Verification items for the finished model (mm, model axes). Give positions to 0.01 mm unless a question says otherwise; leave off trailing zeros. Loops run counter-clockwise (first coordinate to the right, second up) from the corner with the lowest first, then second, coordinate; pieces in that order, holes last. Notation, with made-up numbers: (9.25, 84) - (54.25, 84) arc R15 cw to (54.25, 95) - close; hole circle Ø4 at (14, 42). An arc over 180 degrees is marked (long way). One line per question, with ' | ' between items. Start each with the question number.
1. Thickness scan on line 1 along Y through (x, z) = (170, 0.9); line 2 along Y through (x, z) = (4, 1.7); line 3 along Y through (x, z) = (80, 2.7). Record the ranges inside material, lowest first. Write a range as from..to.
2. Section check B-B, the plane y = 5.5. Enter the section's corners in (x, z), then the cut area to 3 significant figures.
3. Section check C-C, the plane z = 2.2. State how many separate pieces and enclosed holes the cut face has, then the cut area to 3 significant figures.
4. Section check A-A, the plane x = 134.5. Enter the section's corners in (y, z).
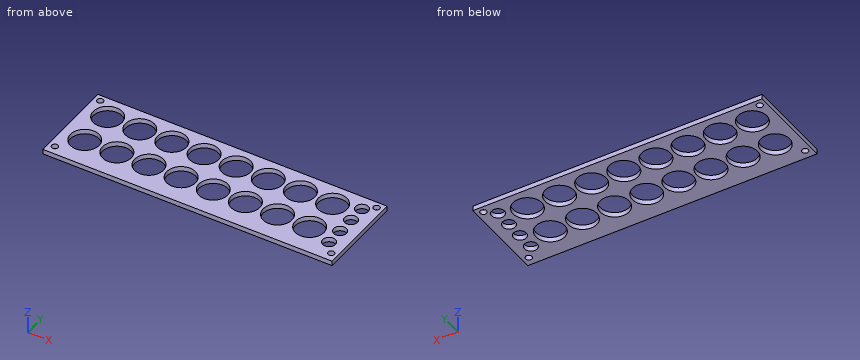
from build123d import *

# Parameters (mm, degrees)
CYLINDER023_R     = 2
CYLINDER023_DEPTH = 3
CYLINDER022_R     = 2
CYLINDER022_DEPTH = 3
CYLINDER021_R     = 2
CYLINDER021_DEPTH = 3
CYLINDER020_R     = 2
CYLINDER020_DEPTH = 3
CYLINDER019_R     = 4
CYLINDER019_DEPTH = 3
CYLINDER018_R     = 4
CYLINDER018_DEPTH = 3
CYLINDER013_R     = 4
CYLINDER013_DEPTH = 3
CYLINDER012_R     = 4
CYLINDER012_DEPTH = 3
CYLINDER017_R     = 9
CYLINDER017_DEPTH = 3
CYLINDER016_R     = 9
CYLINDER016_DEPTH = 3
CYLINDER015_R     = 9
CYLINDER015_DEPTH = 3
CYLINDER014_R     = 9
CYLINDER014_DEPTH = 3
CYLINDER007_R     = 9
CYLINDER007_DEPTH = 3
CYLINDER006_R     = 9
CYLINDER006_DEPTH = 3
CYLINDER005_R     = 9
CYLINDER005_DEPTH = 3
CYLINDER004_R     = 9
CYLINDER004_DEPTH = 3
CYLINDER011_R     = 9
CYLINDER011_DEPTH = 3
CYLINDER010_R     = 9
CYLINDER010_DEPTH = 3
CYLINDER009_R     = 9
CYLINDER009_DEPTH = 3
CYLINDER008_R     = 9
CYLINDER008_DEPTH = 3
CYLINDER003_R     = 9
CYLINDER003_DEPTH = 3
CYLINDER002_R     = 9
CYLINDER002_DEPTH = 3
CYLINDER001_R     = 9
CYLINDER001_DEPTH = 3
CYLINDER_R        = 9
CYLINDER_DEPTH    = 3
BOX_W             = 180
BOX_H             = 55
BOX_DEPTH         = 3


with BuildPart() as cylinder023:
    # Cylinder023 → Cylinder023 (new body)
    with BuildSketch(Plane(origin=(176, 51, 0), x_dir=(1, 0, 0), z_dir=(0, 0, 1))):
        Circle(CYLINDER023_R)
    extrude(amount=CYLINDER023_DEPTH)


with BuildPart() as cylinder022:
    # Cylinder022 → Cylinder022 (new body)
    with BuildSketch(Plane(origin=(4, 51, 0), x_dir=(1, 0, 0), z_dir=(0, 0, 1))):
        Circle(CYLINDER022_R)
    extrude(amount=CYLINDER022_DEPTH)


with BuildPart() as cylinder021:
    # Cylinder021 → Cylinder021 (new body)
    with BuildSketch(Plane(origin=(176, 5.5, 0), x_dir=(1, 0, 0), z_dir=(0, 0, 1))):
        Circle(CYLINDER021_R)
    extrude(amount=CYLINDER021_DEPTH)


with BuildPart() as cylinder020:
    # Cylinder020 → Cylinder020 (new body)
    with BuildSketch(Plane(origin=(4, 5.5, 0), x_dir=(1, 0, 0), z_dir=(0, 0, 1))):
        Circle(CYLINDER020_R)
    extrude(amount=CYLINDER020_DEPTH)


with BuildPart() as cylinder019:
    # Cylinder019 → Cylinder019 (new body)
    with BuildSketch(Plane(origin=(170, 13, 0), x_dir=(1, 0, 0), z_dir=(0, 0, 1))):
        Circle(CYLINDER019_R)
    extrude(amount=CYLINDER019_DEPTH)


with BuildPart() as cylinder018:
    # Cylinder018 → Cylinder018 (new body)
    with BuildSketch(Plane(origin=(170, 24, 0), x_dir=(1, 0, 0), z_dir=(0, 0, 1))):
        Circle(CYLINDER018_R)
    extrude(amount=CYLINDER018_DEPTH)


with BuildPart() as cylinder013:
    # Cylinder013 → Cylinder013 (new body)
    with BuildSketch(Plane(origin=(170, 35, 0), x_dir=(1, 0, 0), z_dir=(0, 0, 1))):
        Circle(CYLINDER013_R)
    extrude(amount=CYLINDER013_DEPTH)


with BuildPart() as cylinder012:
    # Cylinder012 → Cylinder012 (new body)
    with BuildSketch(Plane(origin=(170, 46, 0), x_dir=(1, 0, 0), z_dir=(0, 0, 1))):
        Circle(CYLINDER012_R)
    extrude(amount=CYLINDER012_DEPTH)


with BuildPart() as cylinder017:
    # Cylinder017 → Cylinder017 (new body)
    with BuildSketch(Plane(origin=(154.5, 18.5, 0), x_dir=(1, 0, 0), z_dir=(0, 0, 1))):
        Circle(CYLINDER017_R)
    extrude(amount=CYLINDER017_DEPTH)


with BuildPart() as cylinder016:
    # Cylinder016 → Cylinder016 (new body)
    with BuildSketch(Plane(origin=(134.5, 18.5, 0), x_dir=(1, 0, 0), z_dir=(0, 0, 1))):
        Circle(CYLINDER016_R)
    extrude(amount=CYLINDER016_DEPTH)


with BuildPart() as cylinder015:
    # Cylinder015 → Cylinder015 (new body)
    with BuildSketch(Plane(origin=(114.5, 18.5, 0), x_dir=(1, 0, 0), z_dir=(0, 0, 1))):
        Circle(CYLINDER015_R)
    extrude(amount=CYLINDER015_DEPTH)


with BuildPart() as cylinder014:
    # Cylinder014 → Cylinder014 (new body)
    with BuildSketch(Plane(origin=(94.5, 18.5, 0), x_dir=(1, 0, 0), z_dir=(0, 0, 1))):
        Circle(CYLINDER014_R)
    extrude(amount=CYLINDER014_DEPTH)


with BuildPart() as cylinder007:
    # Cylinder007 → Cylinder007 (new body)
    with BuildSketch(Plane(origin=(74.5, 18.5, 0), x_dir=(1, 0, 0), z_dir=(0, 0, 1))):
        Circle(CYLINDER007_R)
    extrude(amount=CYLINDER007_DEPTH)


with BuildPart() as cylinder006:
    # Cylinder006 → Cylinder006 (new body)
    with BuildSketch(Plane(origin=(54.5, 18.5, 0), x_dir=(1, 0, 0), z_dir=(0, 0, 1))):
        Circle(CYLINDER006_R)
    extrude(amount=CYLINDER006_DEPTH)


with BuildPart() as cylinder005:
    # Cylinder005 → Cylinder005 (new body)
    with BuildSketch(Plane(origin=(34.5, 18.5, 0), x_dir=(1, 0, 0), z_dir=(0, 0, 1))):
        Circle(CYLINDER005_R)
    extrude(amount=CYLINDER005_DEPTH)


with BuildPart() as cylinder004:
    # Cylinder004 → Cylinder004 (new body)
    with BuildSketch(Plane(origin=(14.5, 18.5, 0), x_dir=(1, 0, 0), z_dir=(0, 0, 1))):
        Circle(CYLINDER004_R)
    extrude(amount=CYLINDER004_DEPTH)


with BuildPart() as cylinder011:
    # Cylinder011 → Cylinder011 (new body)
    with BuildSketch(Plane(origin=(154.5, 41.5, 0), x_dir=(1, 0, 0), z_dir=(0, 0, 1))):
        Circle(CYLINDER011_R)
    extrude(amount=CYLINDER011_DEPTH)


with BuildPart() as cylinder010:
    # Cylinder010 → Cylinder010 (new body)
    with BuildSketch(Plane(origin=(134.5, 41.5, 0), x_dir=(1, 0, 0), z_dir=(0, 0, 1))):
        Circle(CYLINDER010_R)
    extrude(amount=CYLINDER010_DEPTH)


with BuildPart() as cylinder009:
    # Cylinder009 → Cylinder009 (new body)
    with BuildSketch(Plane(origin=(114.5, 41.5, 0), x_dir=(1, 0, 0), z_dir=(0, 0, 1))):
        Circle(CYLINDER009_R)
    extrude(amount=CYLINDER009_DEPTH)


with BuildPart() as cylinder008:
    # Cylinder008 → Cylinder008 (new body)
    with BuildSketch(Plane(origin=(94.5, 41.5, 0), x_dir=(1, 0, 0), z_dir=(0, 0, 1))):
        Circle(CYLINDER008_R)
    extrude(amount=CYLINDER008_DEPTH)


with BuildPart() as cylinder003:
    # Cylinder003 → Cylinder003 (new body)
    with BuildSketch(Plane(origin=(74.5, 41.5, 0), x_dir=(1, 0, 0), z_dir=(0, 0, 1))):
        Circle(CYLINDER003_R)
    extrude(amount=CYLINDER003_DEPTH)


with BuildPart() as cylinder002:
    # Cylinder002 → Cylinder002 (new body)
    with BuildSketch(Plane(origin=(54.5, 41.5, 0), x_dir=(1, 0, 0), z_dir=(0, 0, 1))):
        Circle(CYLINDER002_R)
    extrude(amount=CYLINDER002_DEPTH)


with BuildPart() as cylinder001:
    # Cylinder001 → Cylinder001 (new body)
    with BuildSketch(Plane(origin=(34.5, 41.5, 0), x_dir=(1, 0, 0), z_dir=(0, 0, 1))):
        Circle(CYLINDER001_R)
    extrude(amount=CYLINDER001_DEPTH)


with BuildPart() as cylinder:
    # Cylinder → Cylinder (new body)
    with BuildSketch(Plane(origin=(14.5, 41.5, 0), x_dir=(1, 0, 0), z_dir=(0, 0, 1))):
        Circle(CYLINDER_R)
    extrude(amount=CYLINDER_DEPTH)


with BuildPart() as cut023:
    # Box → Box (new body)
    with BuildSketch(Plane.XY):
        with Locations((90, 27.5)):
            Rectangle(BOX_W, BOX_H)
    extrude(amount=BOX_DEPTH)

    # Cut: cut Cylinder
    add(cylinder.part, mode=Mode.SUBTRACT)

    # Cut001: cut Cylinder001
    add(cylinder001.part, mode=Mode.SUBTRACT)

    # Cut002: cut Cylinder002
    add(cylinder002.part, mode=Mode.SUBTRACT)

    # Cut003: cut Cylinder003
    add(cylinder003.part, mode=Mode.SUBTRACT)

    # Cut004: cut Cylinder008
    add(cylinder008.part, mode=Mode.SUBTRACT)

    # Cut005: cut Cylinder009
    add(cylinder009.part, mode=Mode.SUBTRACT)

    # Cut006: cut Cylinder010
    add(cylinder010.part, mode=Mode.SUBTRACT)

    # Cut007: cut Cylinder011
    add(cylinder011.part, mode=Mode.SUBTRACT)

    # Cut008: cut Cylinder004
    add(cylinder004.part, mode=Mode.SUBTRACT)

    # Cut009: cut Cylinder005
    add(cylinder005.part, mode=Mode.SUBTRACT)

    # Cut010: cut Cylinder006
    add(cylinder006.part, mode=Mode.SUBTRACT)

    # Cut011: cut Cylinder007
    add(cylinder007.part, mode=Mode.SUBTRACT)

    # Cut012: cut Cylinder014
    add(cylinder014.part, mode=Mode.SUBTRACT)

    # Cut013: cut Cylinder015
    add(cylinder015.part, mode=Mode.SUBTRACT)

    # Cut014: cut Cylinder016
    add(cylinder016.part, mode=Mode.SUBTRACT)

    # Cut015: cut Cylinder017
    add(cylinder017.part, mode=Mode.SUBTRACT)

    # Cut016: cut Cylinder012
    add(cylinder012.part, mode=Mode.SUBTRACT)

    # Cut017: cut Cylinder013
    add(cylinder013.part, mode=Mode.SUBTRACT)

    # Cut018: cut Cylinder018
    add(cylinder018.part, mode=Mode.SUBTRACT)

    # Cut019: cut Cylinder019
    add(cylinder019.part, mode=Mode.SUBTRACT)

    # Cut020: cut Cylinder020
    add(cylinder020.part, mode=Mode.SUBTRACT)

    # Cut021: cut Cylinder021
    add(cylinder021.part, mode=Mode.SUBTRACT)

    # Cut022: cut Cylinder022
    add(cylinder022.part, mode=Mode.SUBTRACT)

    # Cut023: cut Cylinder023
    add(cylinder023.part, mode=Mode.SUBTRACT)


solid = cut023.part
Results list:
1) line 1: 0..9, 17..20, 28..31, 39..42, 50..55 | line 2: 0..3.5, 7.5..49, 53..55 | line 3: 0..11.38, 25.62..34.38, 48.62..55
2) outline: (0, 0) - (2, 0) - (2, 3) - (0, 3) - close; (6, 0) - (174, 0) - (174, 3) - (6, 3) - close; (178, 0) - (180, 0) - (180, 3) - (178, 3) - close | area: 516 mm²
3) separate pieces: 1 | enclosed holes: 24 | area: 5,580 mm²
4) outline: (0, 0) - (9.5, 0) - (9.5, 3) - (0, 3) - close; (27.5, 0) - (32.5, 0) - (32.5, 3) - (27.5, 3) - close; (50.5, 0) - (55, 0) - (55, 3) - (50.5, 3) - close
